Here's how the part is built. I have some questions about the finished solid (model axes, mm). A direction names the side the tool comes from. Round coordinates to 2 decimals unless told otherwise and drop trailing zeros. One line per question, with ' | ' between items. Start each with the question number.
(1) Will these pins go through, and if not, where does the flat tip stop? pin 1 (7.5 mm diameter, centred on x = -50.8, y = 0, fed in from +Z); pin 2 (12 mm diameter, centred on x = -70, y = 0, fed in from +Z); pin 3 (1.1 mm diameter, centred on x = 42, y = -3, fed in from +Z).
(2) For faces 4 (the flat face through (-15, -16.002, 0)), 5 (the flat face through (-178.591, -0.267, 463.404)), 6 (the flat face through (-107, 16.002, 449)), 7 (the flat face through (-37, 0, 19.05)), which set-ups out of +Z, -Z, +X, -X, +Y, -Y let a thin tool reach every point of the face, with its end or its side?
(3) If I drill on L1, parallel to X at y = 6.5, z = 43; L2, parallel to X at y = 3, z = 374; L3, parallel to Y at x = -50, z = 17, over which ranges is the centre line in solid material (lowest first)?
(4) Thinking about a two-plate mould opening in Y: for faces 1 (the cylindrical face through (-14.91, 15.05, 212.11)), 2 (the cylindrical face through (-142.255, -18.145, 444.884)), 3 (the flat face through (-76.2, -17, 0)), which applies, pulls with the +Y half, pulls with the -Y half, needs draft (parallel to the pull), parting line crosses it, or undercut?
(5) Imagine slicing it at A-A (y = 0). Give the number of separate pieces and of enclosed holes in the cut face, plus the area to 3 significant figures.
from build123d import *
from build123d import SkipClean  # not in build123d's __all__

# Parameters (mm, degrees)
F1_DEPTH       = 44.45
F1_DEPTH_BACK  = 76.2
F5_DEPTH       = 419.1
F5_DEPTH_BACK  = 28.956
F7_DEPTH       = 145.288
F10_DEPTH      = 38.1
F10_DEPTH_BACK = 101.6
F12_DEPTH      = 154.2941466414
F13_R          = 6.35
F14_DEPTH      = 6.35
F15_R          = 6.35
F16_DEPTH      = 6.35


with BuildPart() as f1:
    # F0 (on Right) → F1 (new body, two sides)
    with BuildSketch(Plane.YZ) as f1_sk:
        with BuildLine():
            ThreePointArc((19.05, 15.875), (18.1200640303, 18.1200640303), (15.875, 19.05))
            Line((15.875, 19.05), (-15.875, 19.05))
            ThreePointArc((-15.875, 19.05), (-18.1200640303, 18.1200640303), (-19.05, 15.875))
            Line((-19.05, 15.875), (-19.05, -15.875))
            ThreePointArc((-19.05, -15.875), (-18.1200640303, -18.1200640303), (-15.875, -19.05))
            Line((-15.875, -19.05), (15.875, -19.05))
            ThreePointArc((15.875, -19.05), (18.1200640303, -18.1200640303), (19.05, -15.875))
            Line((19.05, -15.875), (19.05, 15.875))
        make_face()
        with BuildLine():
            Line((-16.002, -12.827), (-16.002, 12.827))
            ThreePointArc((-16.002, 12.827), (-15.0720640303, 15.0720640303), (-12.827, 16.002))
            Line((-12.827, 16.002), (12.827, 16.002))
            ThreePointArc((12.827, 16.002), (15.0720640303, 15.0720640303), (16.002, 12.827))
            Line((16.002, 12.827), (16.002, -12.827))
            ThreePointArc((16.002, -12.827), (15.0720640303, -15.0720640303), (12.827, -16.002))
            Line((12.827, -16.002), (-12.827, -16.002))
            ThreePointArc((-12.827, -16.002), (-15.0720640303, -15.0720640303), (-16.002, -12.827))
        make_face(mode=Mode.SUBTRACT)
    extrude(amount=F1_DEPTH)
    extrude(f1_sk.sketch, amount=-F1_DEPTH_BACK)

    # F4 (on face) → F5 (join, two sides)
    with BuildSketch(Plane(origin=(-8.3589183447, 0, 31.1959079588), x_dir=(0.9659258263, 0, 0.2588190451), z_dir=(0.2588190451, 0, -0.9659258263))) as f5_sk:
        with BuildLine():
            ThreePointArc((44.45, 15.875), (43.5200640303, 18.1200640303), (41.275, 19.05))
            Line((41.275, 19.05), (9.525, 19.05))
            ThreePointArc((9.525, 19.05), (7.2799359697, 18.1200640303), (6.35, 15.875))
            Line((6.35, 15.875), (6.35, -15.875))
            ThreePointArc((6.35, -15.875), (7.2799359697, -18.1200640303), (9.525, -19.05))
            Line((9.525, -19.05), (41.275, -19.05))
            ThreePointArc((41.275, -19.05), (43.5200640303, -18.1200640303), (44.45, -15.875))
            Line((44.45, -15.875), (44.45, 15.875))
        make_face()
        with BuildLine():
            Line((12.573, 16.002), (38.227, 16.002))
            ThreePointArc((38.227, 16.002), (40.4720640303, 15.0720640303), (41.402, 12.827))
            Line((41.402, 12.827), (41.402, -12.827))
            ThreePointArc((41.402, -12.827), (40.4720640303, -15.0720640303), (38.227, -16.002))
            Line((38.227, -16.002), (12.573, -16.002))
            ThreePointArc((12.573, -16.002), (10.3279359697, -15.0720640303), (9.398, -12.827))
            Line((9.398, -12.827), (9.398, 12.827))
            ThreePointArc((9.398, 12.827), (10.3279359697, 15.0720640303), (12.573, 16.002))
        make_face(mode=Mode.SUBTRACT)
    extrude(amount=-F5_DEPTH)
    extrude(f5_sk.sketch, amount=F5_DEPTH_BACK)

    # F6 (on face) → F7 (cut)
    with BuildSketch(Plane(origin=(-76.2, 0, 0), x_dir=(0, -1, 0), z_dir=(-1, 0, 0))):
        with BuildLine():
            Line((12.827, 16.002), (-12.827, 16.002))
            ThreePointArc((-12.827, 16.002), (-15.0720640303, 15.0720640303), (-16.002, 12.827))
            Line((-16.002, 12.827), (-16.002, -12.827))
            ThreePointArc((-16.002, -12.827), (-15.0720640303, -15.0720640303), (-12.827, -16.002))
            Line((-12.827, -16.002), (12.827, -16.002))
            ThreePointArc((12.827, -16.002), (15.0720640303, -15.0720640303), (16.002, -12.827))
            Line((16.002, -12.827), (16.002, 12.827))
            ThreePointArc((16.002, 12.827), (15.0720640303, 15.0720640303), (12.827, 16.002))
        make_face()
    with SkipClean():  # cleaning this boolean's faces spoils the solid; the shape is the same uncleaned
        extrude(amount=-F7_DEPTH, mode=Mode.SUBTRACT)

    # F9 (on face) → F10 (join, two sides)
    with BuildSketch(Plane(origin=(-232.1066250318, 0, 108.2330967608), x_dir=(0, 1, 0), z_dir=(0.906307787, 0, -0.4226182617))) as f10_sk:
        with BuildLine():
            ThreePointArc((19.05, 377.0523048448), (18.1200640303, 379.297368875), (15.875, 380.2273048448))
            Line((15.875, 380.2273048448), (-15.875, 380.2273048448))
            ThreePointArc((-15.875, 380.2273048448), (-18.1200640303, 379.297368875), (-19.05, 377.0523048448))
            Line((-19.05, 377.0523048448), (-19.05, 345.3023048448))
            ThreePointArc((-19.05, 345.3023048448), (-18.1200640303, 343.0572408145), (-15.875, 342.1273048448))
            Line((-15.875, 342.1273048448), (15.875, 342.1273048448))
            ThreePointArc((15.875, 342.1273048448), (18.1200640303, 343.0572408145), (19.05, 345.3023048448))
            Line((19.05, 345.3023048448), (19.05, 377.0523048448))
        make_face()
        with BuildLine():
            Line((-12.827, 377.1793048448), (12.827, 377.1793048448))
            ThreePointArc((12.827, 377.1793048448), (15.0720640303, 376.249368875), (16.002, 374.0043048448))
            Line((16.002, 374.0043048448), (16.002, 348.3503048448))
            ThreePointArc((16.002, 348.3503048448), (15.0720640303, 346.1052408145), (12.827, 345.1753048448))
            Line((12.827, 345.1753048448), (-12.827, 345.1753048448))
            ThreePointArc((-12.827, 345.1753048448), (-15.0720640303, 346.1052408145), (-16.002, 348.3503048448))
            Line((-16.002, 348.3503048448), (-16.002, 374.0043048448))
            ThreePointArc((-16.002, 374.0043048448), (-15.0720640303, 376.249368875), (-12.827, 377.1793048448))
        make_face(mode=Mode.SUBTRACT)
    with SkipClean():  # cleaning this boolean's faces spoils the solid; the shape is the same uncleaned
        extrude(amount=F10_DEPTH)
        extrude(f10_sk.sketch, amount=-F10_DEPTH_BACK)

    # F11 (on face) → F12 (cut, through all)
    with BuildSketch(Plane(origin=(-197.5762983457, 0, 92.1313409885), x_dir=(0, 1, 0), z_dir=(0.906307787, 0, -0.4226182617))):
        with BuildLine():
            ThreePointArc((-12.827, 377.1793048448), (-15.0720640303, 376.249368875), (-16.002, 374.0043048448))
            Line((-16.002, 374.0043048448), (-16.002, 348.3503048448))
            ThreePointArc((-16.002, 348.3503048448), (-15.0720640303, 346.1052408145), (-12.827, 345.1753048448))
            Line((-12.827, 345.1753048448), (12.827, 345.1753048448))
            ThreePointArc((12.827, 345.1753048448), (15.0720640303, 346.1052408145), (16.002, 348.3503048448))
            Line((16.002, 348.3503048448), (16.002, 374.0043048448))
            ThreePointArc((16.002, 374.0043048448), (15.0720640303, 376.249368875), (12.827, 377.1793048448))
            Line((12.827, 377.1793048448), (-12.827, 377.1793048448))
        make_face()
    with SkipClean():  # cleaning this boolean's faces spoils the solid; the shape is the same uncleaned
        extrude(amount=-F12_DEPTH, mode=Mode.SUBTRACT)

    # F13 (on face) → F14 (cut)
    with BuildSketch(Plane.XY.offset(19.05)):
        with Locations((-50.8, 0)):
            Circle(F13_R)
    with SkipClean():  # cleaning this boolean's faces spoils the solid; the shape is the same uncleaned
        extrude(amount=-F14_DEPTH, mode=Mode.SUBTRACT)

    # F15 (on face) → F16 (cut)
    with BuildSketch(Plane(origin=(144.5892468675, 0, 310.0726405387), x_dir=(0.906307787, 0, -0.4226182617), z_dir=(-0.4226182617, 0, -0.906307787))):
        with Locations((-332.301324905, 0)):
            Circle(F15_R)
    with SkipClean():  # cleaning this boolean's faces spoils the solid; the shape is the same uncleaned
        extrude(amount=-F16_DEPTH, mode=Mode.SUBTRACT)


solid = f1.part
Check sheet entries:
1) pin 1: z = 444.97 | pin 2: z = 454.97 | pin 3: z = 19.05
2) face 4: +X, -X | face 5: +Z, -X, +Y, -Y | face 6: none | face 7: -X, +Y, -Y
3) L1: -4.95 to -1.79, 31.34 to 34.5 | L2: -93.64 to -90.48, -57.35 to -54.19 | L3: -18.84 to -6.3, 6.3 to 18.84
4) face 1: undercut | face 2: pulls with the -Y half | face 3: needs draft
5) separate pieces: 5 | enclosed holes: 1 | area: 4,020 mm^2
